```python
from build123d import *

# Parameters (mm, degrees)
SKETCH4_OUTSIDE_W  = 22.844
SKETCH4_OUTSIDE_H  = 22.844
CUT_EXTRUDE1_DEPTH = 37.85314377


with BuildPart() as part:
    # Sketch3 → Revolve1 (revolve)
    with BuildSketch(Plane(origin=(0, 0, 0), x_dir=(0, 0, -1), z_dir=(1, 0, 0)), mode=Mode.PRIVATE) as revolve1_sk:
        Polygon((17.859375, 2.2225), (17.859375, 0), (-17.859375, 0), (-17.859375, 5.55625), (-17.363110767, 6.415804866), (-13.890625, 6.415804866), (-13.890625, 3.175), (16.906875, 3.175), align=None)
    revolve(revolve1_sk.sketch.rotate(Axis((0, 0, 17.859375), (0, 0, -1)), 90), axis=Axis((0, 0, 17.859375), (0, 0, -1)))

    # Sketch4 outside → Cut-Extrude1 (cut, through all)
    with BuildSketch(Plane.XY.offset(17.859375)):
        Rectangle(SKETCH4_OUTSIDE_W, SKETCH4_OUTSIDE_H)
        Polygon((5.55625, -3.207902433), (5.55625, 3.207902433), (0, 6.415804866), (-5.55625, 3.207902433), (-5.55625, -3.207902433), (0, -6.415804866), align=None, mode=Mode.SUBTRACT)
    extrude(amount=-CUT_EXTRUDE1_DEPTH, mode=Mode.SUBTRACT)


solid = part.part
```
The listing builds one solid part. Answer for the finished solid, in the listing's coordinates (mm). A direction names the side the tool comes from. Coordinates: 2 decimals unless noted, no trailing zeros. Write each loop counter-clockwise with the first axis right and the second up, starting at its lowest first coordinate (ties: lowest second). Pieces come first, ordered by that corner, then holes.
Q1. Which of the six approach directions +Z, -Z, +X, -X, +Y, -Y give full straight-line access (tool end or side, diameter ignored) to faces 1 (the flat face through (2.739, -4.834, 15.903)), 2 (the flat face through (-3, 3, 13.891))?
Returned:
face 1: +Z, -Z, +X, -Y
face 2: -Z
Q2. Section A-A, the plane z = 16 is taken. Write down the section's boundary in (x, y).
Returned:
outline: (-5.56, -3.21) - (0, -6.42) - (5.56, -3.21) - (5.56, 3.21) - (0, 6.42) - (-5.56, 3.21) - close
Q3. Find the intervals of material crossed by line 1 along Z through (x, y) = (1.5, 3.25); line 2 along Y through (x, z) = (0, 13) (3 decimals); line 3 along X through (y, z) = (1.25, -12), in increasing order.
Returned:
line 1: z = 13.89 to 17.86
line 2: y = -3.175 to 3.175
line 3: x = -2.92 to 2.92
Q4. Section B-B, the plane z = -8.5 is taken. Write down the section's boundary in (x, y) (3 decimals).
Returned:
outline: circle Ø6.35 at (0, 0)
Q5. Given P1, Ø3, axis at x = -3, y = -4, coming from the -Z side; P2, Ø3.5, axis at x = -2.5, y = -0.5, coming from the -Z side; P3, Ø1, axis at x = 2, z = 9, coming from the -Y side; P4, Ø5, axis at x = -1.5, z = -11, coming from the +Y side (3 decimals), each flat-ended and moving along its own axis, determine where each tip first touches the part or whether it passes through.
Returned:
P1: stops at z = 13.89
P2: stops at z = -17.86
P3: stops at y = -2.8
P4: stops at y = 3.175
